Here's how the part is built. I have some questions about the finished solid (model axes, mm). Face numbers are marked on the shaded views. A direction names the side the tool comes from. Give positions to 0.01 mm unless a question says otherwise; leave off trailing zeros. Loops run counter-clockwise (first coordinate to the right, second up) from the corner with the lowest first, then second, coordinate; pieces in that order, holes last. Notation, with made-up numbers: (48, 19) - (75, 19) arc R20 cw to (75, 58) - close; hole circle Ø7 at (9.5, 88.25). An arc over 180 degrees is marked (long way). Return JSON: item names as keys, results as strings. Group by question number.
(1) On a 3-axis mill with a long thin cutter (end or side, diameter ignored), from which of +Z, -Z, +X, -X, +Y, -Y can I reach the whole of each face in a straight line? I mean the marked faces 5 and 6. Say none if no direction works.
(2) I need wall thicknesses on probe 1 along Y at (x, z) = (4, 14); probe 2 along Z at (x, y) = (-0.25, 6); probe 3 along Z at (x, y) = (1, -3). Which ranges of each line are inside material? Lowest first, please. Write a range as [from, to].
(3) If we section it at A-A (z = 22): Please give me the cut outline in (x, y), then the cut area to 3 significant figures.
(4) If we section it at D-D (z = 9.5): Please give me the cut outline in (x, y), then the cut area to 3 significant figures.
(5) If we section it at B-B (y = -5.5): Please give me the cut outline in (x, z), then the cut area to 3 significant figures.
(6) If we section it at C-C (x = 0): Please give me the cut outline in (y, z).
(7) If we mould it in two halves opening along Y, with no side actions, what happens to the marked faces 1, 2, 3 and 4? For each: released by +Y, released by -Y, zero draft, split by the parting line, or undercut.
(8) For P1, Ø6, axis at y = 2.5, z = 10.5, coming from the -X side; P2, Ø5.5, axis at x = 2, y = -0.5, coming from the +Z side; P3, Ø1.5, axis at y = 4.5, z = 34, coming from the +X side, each with a flat end and sliding along its axis, tell me the tip position at first contact or that it passes through.
```python
from build123d import *

# Parameters (mm, degrees)
F0_W     = 25.4
F0_H     = 15
F1_DEPTH = 38
F2_W     = 7
F2_H     = 33
F3_DEPTH = 25.4
F4_R     = 5
F5_R     = 3.25
F6_DEPTH = 25


with BuildPart() as f1:
    # F0 (on Top) → F1 (new body)
    with BuildSketch(Plane.XY):
        Rectangle(F0_W, F0_H)
    extrude(amount=F1_DEPTH)

    # F2 (on face) → F3 (cut, through all)
    with BuildSketch(Plane.YZ.offset(12.7)):
        with Locations((0, 21.5)):
            Rectangle(F2_W, F2_H)
    extrude(amount=-F3_DEPTH, mode=Mode.SUBTRACT)

    # F4
    f4_edges = [f1.edges().sort_by_distance(p)[0] for p in [
        (12.7, 5.5, 38),
        (12.7, -5.5, 38),
        (-12.7, -5.5, 38),
        (-12.7, 5.5, 38),
    ]]
    fillet(f4_edges, radius=F4_R)

    # F5 (on face) → F6 (cut)
    with BuildSketch(Plane.XZ.offset(7.5)):
        with Locations((0, 22)):
            Circle(F5_R)
    extrude(amount=-F6_DEPTH, mode=Mode.SUBTRACT)


solid = f1.part
```
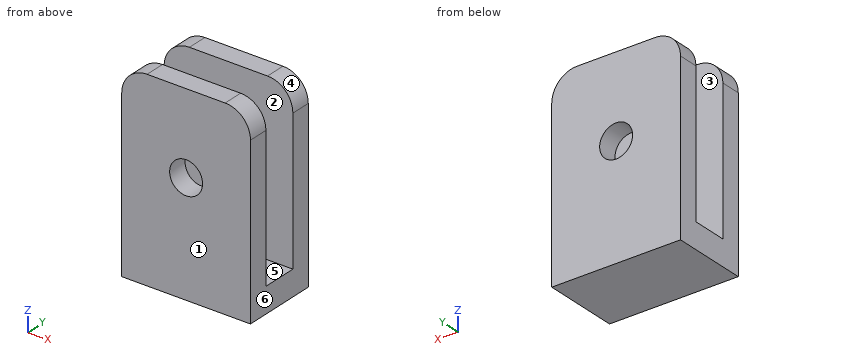
Values:
{
 "1": {"face 5": "+Z, +X, -X", "face 6": "+Z, -Z, +X, +Y, -Y"},
 "2": {"probe 1": "[-7.5, -3.5], [3.5, 7.5]", "probe 2": "[0, 18.76], [25.24, 38]", "probe 3": "[0, 5]"},
 "3": {"outline": "(-12.7, -7.5) - (-3.25, -7.5) - (-3.25, -3.5) - (-12.7, -3.5) - close; (-12.7, 3.5) - (-3.25, 3.5) - (-3.25, 7.5) - (-12.7, 7.5) - close; (3.25, -7.5) - (12.7, -7.5) - (12.7, -3.5) - (3.25, -3.5) - close; (3.25, 3.5) - (12.7, 3.5) - (12.7, 7.5) - (3.25, 7.5) - close", "area": "151 mm2"},
 "4": {"outline": "(-12.7, -7.5) - (12.7, -7.5) - (12.7, -3.5) - (-12.7, -3.5) - close; (-12.7, 3.5) - (12.7, 3.5) - (12.7, 7.5) - (-12.7, 7.5) - close", "area": "203 mm2"},
 "5": {"outline": "(-12.7, 0) - (12.7, 0) - (12.7, 33) arc R5 ccw to (7.7, 38) - (-7.7, 38) arc R5 ccw to (-12.7, 33) - close; hole circle Ø6.5 at (0, 22)", "area": "921 mm2"},
 "6": {"outline": "(-7.5, 0) - (7.5, 0) - (7.5, 18.75) - (3.5, 18.75) - (3.5, 5) - (-3.5, 5) - (-3.5, 18.75) - (-7.5, 18.75) - close; (-7.5, 25.25) - (-3.5, 25.25) - (-3.5, 38) - (-7.5, 38) - close; (3.5, 25.25) - (7.5, 25.25) - (7.5, 38) - (3.5, 38) - close"},
 "7": {"face 1": "released by -Y", "face 2": "undercut", "face 3": "undercut", "face 4": "zero draft"},
 "8": {"P1": "x = -12.7", "P2": "z = 5", "P3": "x = 12.69"}
}
